Autodesk Inventor part; units mm, degrees
ref_plane "YZ Plane" through (0, 0, 0) normal (1, 0, 0) x (0, 1, 0)
ref_plane "XZ Plane" through (0, 0, 0) normal (0, 1, 0) x (-1, 0, 0)
ref_plane "XY Plane" through (0, 0, 0) normal (0, 0, 1) x (1, 0, 0)
sketch "main" plane through (0, 0, 0) normal (0, 0, 1) x (1, 0, 0)
  circle A0 centre (33.3097, -13.5548) radius 2.1844
  arc A1 (33.2126, -19.9041) -> (39.6597, -13.5466) centre (33.3097, -13.5548) ccw
  arc A2 (41.7862, 8.9717) -> (29.1145, 9.6144) centre (35.4643, 9.5687) ccw
  line L0 (39.6597, -13.5466) -> (41.7862, 8.9717)
  line L1 (-68.2903, -7.2251) -> (16.3844, -7.2251)
  line L2 (29.0841, 5.3837) -> (29.1145, 9.6144)
  arc A3 (16.3844, -7.2251) -> (29.0841, 5.3837) centre (16.3844, 5.4749) ccw
  circle A4 centre (35.4643, 9.5687) radius 2.0955
  line L3 (33.4068, -19.9041) -> (-67.7743, -19.9041)
  circle A5 centre (-68.2903, -13.5751) radius 2.1844
  circle A6 centre (-17.4821, -13.5224) radius 2.1844
  arc A7 (-68.2903, -7.2251) -> (-67.7743, -19.9041) centre (-68.2903, -13.5751) ccw
  point P0 (20.4908, -8.19)
  dimension "d0" = 12.7
  dimension "d1" = 12.7
  dimension "d2" = 12.7
  dimension "d3" = 4.191
  dimension "d7" = 4.3688
  dimension "d8" = 4.3688
  dimension "d9" = 12.7
sketch "Sketch1" plane through (0, 0, 0) normal (1, 0, 0) x (0, 1, 0)
  circle A0 centre (-0.0052, 63.4918) radius 2.1844
  arc A1 (6.3442, 63.3994) -> (-0.0181, 69.8418) centre (-0.0052, 63.4918) ccw
  arc A2 (-22.538, 71.9516) -> (-23.1712, 59.2794) centre (-23.1303, 65.6293) ccw
  line L0 (-0.0181, 69.8418) -> (-22.538, 71.9516)
  line L1 (-6.2598, -38.1129) -> (-6.3224, 46.5618)
  line L2 (-18.9405, 59.2522) -> (-23.1712, 59.2794)
  arc A3 (-6.3224, 46.5618) -> (-18.9405, 59.2522) centre (-19.0224, 46.5524) ccw
  circle A4 centre (-23.1303, 65.6293) radius 2.0955
  line L3 (6.344, 63.5936) -> (6.4188, -37.5875)
  circle A5 centre (0.0902, -38.1082) radius 2.1844
  circle A6 centre (0, 12.7) radius 2.1844
  arc A7 (-6.2598, -38.1129) -> (6.4188, -37.5875) centre (0.0902, -38.1082) ccw
  point P0 (0, 0)
extrude "Extrusion1" add sketch "Sketch1" along normal blind 1.5875
equation "\"BendRadius\" = Thickness"
equation "\"BendReliefWidth\" = Thickness"
equation "\"BendReliefDepth\" = 0.5 * Thickness"
equation "\"CornerReliefSize\" = 4 * Thickness"
equation "\"MinimumRemnant\" = 2 * Thickness"
equation "\"TransitionRadius\" = BendRadius"
equation "\"JacobiRadiusSize\" = BendRadius"
equation "\"GapSize\" = Thickness"
properties part number "Passive Gusset" material "Acetal Resin, White"
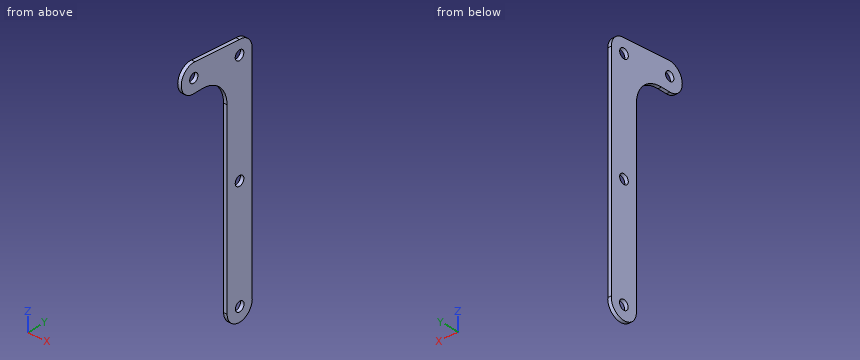
Source: CAD feature listing. Evaluate the final solid. Frame: model axes, mm. Round coordinates to 2 decimals unless told otherwise and drop trailing zeros. Order: outer loops, then holes, each group sorted by start corner. A loop starts at its lowest first (then second) coordinate and runs counter-clockwise, first axis right, second up. Notation, with made-up numbers: (62.5, -29) - (90.5, -29) arc R24 cw to (90.5, -3) - close; hole circle Ø4 at (18.25, 29.25). An arc over 180 degrees is marked (long way). Use a Markdown table: item, result. Add a question column.
1. Section query B-B (z = 12.7). Return the cut outline in (x, y).
2. Section query A-A (x = 0.65). Return the cut outline in (y, z).
3. Section query C-C (y = -5). Return the cut outline in (x, z).
4. Line query: probe 1 along Z at (x, y) = (0.7, 0.5); probe 2 along Y at (x, z) = (1.35, 64.5); probe 3 along Z at (x, y) = (0.2, 2). Output: solid intervals per line, ascending.
5. Section query D-D (z = -13). Return the cut outline in (x, y), then the cut area to 3 significant figures.
6. First-contact query: pin 1 (4 mm diameter, centred on y = 0.09, z = -38.11, fed in from -X). Flat tip, straight axial feed; report the tip coordinate or a pass-through.
Derived:
| question | item | result |
|---|---|---|
| 1 | outline | (0, -6.3) - (1.59, -6.3) - (1.59, -2.18) - (0, -2.18) - close; (0, 2.18) - (1.59, 2.18) - (1.59, 6.38) - (0, 6.38) - close |
| 2 | outline | (-23.17, 59.28) - (-18.94, 59.25) arc R12.7 cw to (-6.32, 46.56) - (-6.26, -38.11) arc R6.35 ccw (long way) to (6.42, -37.59) - (6.34, 63.4) arc R6.35 ccw to (-0.02, 69.84) - (-22.54, 71.95) arc R6.35 ccw (long way) to start; hole circle Ø4.19 at (-23.13, 65.63); hole circle Ø4.37 at (-0.01, 63.49); hole circle Ø4.37 at (0, 12.7); hole circle Ø4.37 at (0.09, -38.11) |
| 3 | outline | (0, -41.9) - (1.59, -41.9) - (1.59, 70.31) - (0, 70.31) - close |
| 4 | probe 1 | -44.44 to -40.25, -35.96 to 10.57, 14.83 to 61.37, 65.62 to 69.82 |
| 4 | probe 2 | -29.38 to -24.9, -21.37 to -1.94, 1.93 to 6.26 |
| 4 | probe 3 | -44.16 to -39.17, -37.05 to 11.82, 13.58 to 62.63, 64.36 to 69.52 |
| 5 | outline | (0, -6.28) - (1.59, -6.28) - (1.59, 6.4) - (0, 6.4) - close |
| 5 | area | 20.1 mm2 |
| 6 | pin 1 | through |
